Design review of the part built by this model. Coordinates are the model's own, in mm. A direction names the side the tool comes from. Round coordinates to 2 decimals unless told otherwise and drop trailing zeros. Order: outer loops, then holes, each group sorted by start corner. A loop starts at its lowest first (then second) coordinate and runs counter-clockwise, first axis right, second up. Notation, with made-up numbers: (83, 35) - (117, 35) arc R23 ccw to (117, 54) - close; hole circle Ø6 at (-2, 65.25). An arc over 180 degrees is marked (long way). Use CSV: the item, a comma, the result in double quotes.
Autodesk Inventor part; units mm, degrees
ref_plane "YZ Plane" through (0, 0, 0) normal (1, 0, 0) x (0, 1, 0)
ref_plane "XZ Plane" through (0, 0, 0) normal (0, 1, 0) x (-1, 0, 0)
ref_plane "XY Plane" through (0, 0, 0) normal (0, 0, 1) x (1, 0, 0)
sketch "스케치1" plane through (0, 0, 0) normal (0, 1, 0) x (-1, 0, 0)
  line L0 (-24.9446, -24.9446) -> (24.9446, -24.9446)
  line L1 (24.9446, -24.9446) -> (24.9446, 24.9446)
  line L2 (24.9446, 24.9446) -> (-24.9446, 24.9446)
  line L3 (-24.9446, 24.9446) -> (-24.9446, -24.9446)
  line L4 (-24.9446, -24.9446) -> (24.9446, 24.9446) construction
  line L5 (24.9446, -24.9446) -> (-24.9446, 24.9446) construction
  line L6 (-28.1446, -28.1446) -> (28.1446, -28.1446)
  line L7 (28.1446, -28.1446) -> (28.1446, 28.1446)
  line L8 (28.1446, 28.1446) -> (-28.1446, 28.1446)
  line L9 (-28.1446, 28.1446) -> (-28.1446, -28.1446)
  line L10 (-28.1446, -28.1446) -> (28.1446, 28.1446) construction
  line L11 (28.1446, -28.1446) -> (-28.1446, 28.1446) construction
  point P0 (0, 0)
  dimension "d0" = 70.554
  dimension "d1" = 3.2
extrude "돌출1" add sketch "스케치1" along normal blind 4.4 contours L3 L2 L1 L0 | L9 L8 L7 L6
sketch "스케치2" plane through (0, 4.4, 0) normal (0, 1, 0) x (1, 0, 0)
  line L0 (-28.1446, 28.1446) -> (-28.1446, -28.1446)
  line L1 (-28.1446, -28.1446) -> (28.1446, -28.1446)
  line L2 (28.1446, -28.1446) -> (28.1446, 28.1446)
  line L3 (28.1446, 28.1446) -> (-28.1446, 28.1446)
  line L4 (26.5446, 26.5446) -> (-26.5446, 26.5446)
  line L5 (-26.5446, 26.5446) -> (-26.5446, -26.5446)
  line L6 (-26.5446, -26.5446) -> (26.5446, -26.5446)
  line L7 (26.5446, -26.5446) -> (26.5446, 26.5446)
  line L8 (26.5446, 26.5446) -> (-26.5446, -26.5446) construction
  line L9 (-26.5446, 26.5446) -> (26.5446, -26.5446) construction
  line L10 (24.5446, 24.5446) -> (-24.5446, 24.5446)
  line L11 (-24.5446, 24.5446) -> (-24.5446, -24.5446)
  line L12 (-24.5446, -24.5446) -> (24.5446, -24.5446)
  line L13 (24.5446, -24.5446) -> (24.5446, 24.5446)
  line L14 (24.5446, 24.5446) -> (-24.5446, -24.5446) construction
  line L15 (-24.5446, 24.5446) -> (24.5446, -24.5446) construction
  point P0 (0, 0)
  point P1 (0, 28.1446)
  point P2 (-28.1446, 0)
  dimension "d4" = 1.6
  dimension "d5" = 2
extrude "돌출2" cut sketch "스케치2" against normal blind 1.2 contours L7 L6 L5 L4 | L13 L12 L11 L10
sketch "스케치3" plane through (0, 3.2, 0) normal (0, 1, 0) x (1, 0, 0)
  line L0 (24.5446, 24.5446) -> (-24.5446, 24.5446)
  line L1 (-24.5446, 24.5446) -> (-24.5446, -24.5446)
  line L2 (-24.5446, -24.5446) -> (24.5446, -24.5446)
  line L3 (24.5446, -24.5446) -> (24.5446, 24.5446)
  line L4 (24.5446, 24.5446) -> (-24.5446, -24.5446) construction
  line L5 (-24.5446, 24.5446) -> (24.5446, -24.5446) construction
  line L6 (-26.5446, -26.5446) -> (-26.5446, 26.5446)
  point P0 (0, 0)
  dimension "d8" = 2
extrude "돌출3" add sketch "스케치3" along normal blind 0.6
sketch "스케치4" plane through (0, 0, 0) normal (0, -1, 0) x (1, 0, 0)
  line L0 (-10, 7.5) -> (10, 7.5)
  line L1 (10, 7.5) -> (10, 2.5)
  line L2 (10, 2.5) -> (-10, 2.5)
  line L3 (-10, 2.5) -> (-10, 7.5)
  line L4 (-10, 7.5) -> (10, 2.5) construction
  line L5 (10, 7.5) -> (-10, 2.5) construction
  line L6 (-10, -2.5) -> (10, -2.5)
  line L7 (10, -2.5) -> (10, -7.5)
  line L8 (10, -7.5) -> (-10, -7.5)
  line L9 (-10, -7.5) -> (-10, -2.5)
  line L10 (-10, -2.5) -> (10, -7.5) construction
  line L11 (10, -2.5) -> (-10, -7.5) construction
  point P0 (0, 0)
  point P1 (0, 5)
  point P2 (0, -5)
  dimension "d11" = 5
  dimension "d12" = 5
  dimension "d13" = 20
  dimension "d14" = 20
  dimension "d15" = 5
  dimension "d16" = 2.5
extrude "돌출4" add sketch "스케치4" along normal blind 10
sketch "스케치5" plane through (-10, 0, 7.5) normal (0, 0, 1) x (1, 0, 0)
  circle A0 centre (15, -5) radius 1.25
  circle A1 centre (5, -5) radius 1.25
  line L0 (-18.1446, 0) -> (38.1446, 0)
  line L1 (0, 0) -> (0, -10)
  point P0 (10, 0)
  dimension "d19" = 2.5
  dimension "d20" = 2.5
  dimension "d21" = 10
  dimension "d22" = 5
  dimension "d23" = 5
extrude "돌출5" cut sketch "스케치5" against normal up to surface (15 mm away)
fillet "모깎기1" radius 1.2 8 edges at (0, 4.4, 28.1446) (28.1446, 4.4, 0) (0, 4.4, -28.1446) (-28.1446, 4.4, 0) (-28.1446, 0, 0) (0, 0, 28.1446) (28.1446, 0, 0) (0, 0, -28.1446)
properties part number "OV-PAM_n_4_bottom"
1) We need section D-D (x = 11). Give the boundary of the cut face in (y, z), then the cut area to 3 significant figures.
Data:
outline,"(0, -26.94) arc R1.2 ccw to (1.2, -28.14) - (3.2, -28.14) arc R1.2 ccw to (4.4, -26.94) - (4.4, -26.54) - (3.2, -26.54) - (3.2, -24.54) - (3.8, -24.54) - (3.8, 24.54) - (3.2, 24.54) - (3.2, 26.54) - (4.4, 26.54) - (4.4, 26.94) arc R1.2 ccw to (3.2, 28.14) - (1.2, 28.14) arc R1.2 ccw to (0, 26.94) - close"
area,"212 mm2"
2) We need section B-B (y = -7.5). Give the boundary of the cut face in (x, z).
Data:
outline,"(-10, -7.5) - (10, -7.5) - (10, -2.5) - (-10, -2.5) - close; (-10, 2.5) - (10, 2.5) - (10, 7.5) - (-10, 7.5) - close"
3) The part is to be moulded in two halves that separate along Y. For faces 1 (the face through (0, 0, 0)), 2 (the face through (4.73, -6.22, -4.96)), 3 (the face through (0, -5, 7.5)), say which applies: +Y half, -Y half, draft (parallel to the pull), parting line (faces both ways), or undercut.
Data:
face 1,"-Y half"
face 2,"undercut"
face 3,"draft"
4) Insertion check: pin 1 Ø1 at (x, y) = (-7, -8.5) entering from -Z; pin 2 Ø6 at (x, y) = (6, -5) entering from +Z; pin 3 Ø4 at (y, z) = (-4.5, 4) entering from +X; pin 4 Ø2 at (x, y) = (-5, -5) entering from -Z. Each pin has a flat end and moves straight along its axis. Give the tip position at first contact, or say it passes through.
Data:
pin 1,"stops at z = -7.5"
pin 2,"stops at z = 7.5"
pin 3,"stops at x = 10"
pin 4,"passes through"
5) We need section C-C (z = 4.5). Give the boundary of the cut face in (x, y), then the cut area to 3 significant figures.
Data:
outline,"(-28.14, 1.2) arc R1.2 ccw to (-26.94, 0) - (-10, 0) - (-10, -10) - (10, -10) - (10, 0) - (26.94, 0) arc R1.2 ccw to (28.14, 1.2) - (28.14, 3.2) arc R1.2 ccw to (26.94, 4.4) - (26.54, 4.4) - (26.54, 3.2) - (24.54, 3.2) - (24.54, 3.8) - (-24.54, 3.8) - (-24.54, 3.2) - (-26.54, 3.2) - (-26.54, 4.4) - (-26.94, 4.4) arc R1.2 ccw to (-28.14, 3.2) - close; hole circle Ø2.5 at (-5, -5); hole circle Ø2.5 at (5, -5)"
area,"402 mm2"
6) To check wall thickness, follow L1, parallel to Y at x = -5, z = 4.6; L2, parallel to Z at x = -7, y = -3.5; L3, parallel to X at y = -4, z = -7. State the ranges of each line that lie inside material, in increasing order. Write a range as from..to.
Data:
L1,"y = -10..-6.25, -3.75..3.8"
L2,"z = -7.5..-2.5, 2.5..7.5"
L3,"x = -10..-5.75, -4.25..4.25, 5.75..10"
7) We need section A-A (x = -5). Give the number of separate pieces and of enclosed holes in the cut face, then the cut area to 3 significant figures.
Data:
separate pieces,"3"
enclosed holes,"0"
area,"287 mm2"
8) For faces 4 (the face through (0, -5, -7.5)), 5 (the face through (0, -5, -2.5)), 6 (the face through (-10, -5, -5)), 7 (the face through (0, 2, 28.145)), 8 (the face through (10, -5, 5)), list the 3-axis set-ups (+Z, -Z, +X, -X, +Y, -Y) from which the entire face can be reached by the end or side of a thin tool; tool diameter is ignored.
Data:
face 4,"-Z, +X, -X, -Y"
face 5,"+X, -X, -Y"
face 6,"+Z, -Z, -X, -Y"
face 7,"+Z, +X, -X, +Y, -Y"
face 8,"+Z, -Z, +X, -Y"
